```python
from build123d import *

# Parameters (mm, degrees)
BOSS_EXTRUDE1_DEPTH = 50.8
SKETCH2_W           = 479.425
SKETCH2_H           = 271.4625
CUT_EXTRUDE1_DEPTH  = 6.35
CUT_EXTRUDE2_DEPTH  = 762
SKETCH6_W           = 198.4375
SKETCH6_H           = 164.295373215
CUT_EXTRUDE3_DEPTH  = 10.922


with BuildPart() as part:
    # Sketch1 → Boss-Extrude1 (new body)
    with BuildSketch(Plane.XY):
        with BuildLine():
            Line((-255.5875, -170.65625), (255.5875, -170.65625))
            ThreePointArc((255.5875, -170.65625), (269.057884182, -165.076634182), (274.6375, -151.60625))
            Line((274.6375, -151.60625), (274.6375, 151.60625))
            ThreePointArc((274.6375, 151.60625), (269.057884182, 165.076634182), (255.5875, 170.65625))
            Line((255.5875, 170.65625), (-255.5875, 170.65625))
            ThreePointArc((-255.5875, 170.65625), (-269.057884182, 165.076634182), (-274.6375, 151.60625))
            Line((-274.6375, 151.60625), (-274.6375, -151.60625))
            ThreePointArc((-274.6375, -151.60625), (-269.057884182, -165.076634182), (-255.5875, -170.65625))
        make_face()
    extrude(amount=-BOSS_EXTRUDE1_DEPTH)

    # Sketch2 → Cut-Extrude1 (cut)
    with BuildSketch(Plane.XY):
        Rectangle(SKETCH2_W, SKETCH2_H)
    extrude(amount=-CUT_EXTRUDE1_DEPTH, mode=Mode.SUBTRACT)

    # Sketch4 → Cut-Extrude2 (cut)
    with BuildSketch(Plane(origin=(274.6375, 0, 0), x_dir=(0, 0, -1), z_dir=(1, 0, 0))):
        with BuildLine():
            Line((50.8, 151.60625), (24.619980511, 151.60625))
            add(Edge.make_bspline(
                [(24.619980511, 151.60625), (37.620188453, 124.390887767), (37.919518366, 93.154889178), (39.820271532, 62.244773812)],
                knots=[0.12550099, 0.12550099, 0.12550099, 0.12550099, 0.642402298, 0.642402298, 0.642402298, 0.642402298], degree=3))
            ThreePointArc((39.820271532, 62.244773812), (41.808148642, 58.008646197), (46.158299596, 56.284517648))
            Line((46.158299596, 56.284517648), (50.8, 56.284517648))
            Line((50.8, 56.284517648), (50.8, 151.60625))
        make_face()
        with BuildLine():
            Line((50.8, 170.65625), (12.7, 170.65625))
            add(Edge.make_bspline(
                [(12.7, 170.65625), (17.558504138, 164.584737247), (21.463596597, 158.21400058), (24.619980511, 151.60625)],
                knots=[0, 0, 0, 0, 0.12550099, 0.12550099, 0.12550099, 0.12550099], degree=3))
            Line((24.619980511, 151.60625), (50.8, 151.60625))
            Line((50.8, 151.60625), (50.8, 170.65625))
        make_face()
        with BuildLine():
            Line((50.8, -96.115482352), (50.8, -170.65625))
            Line((50.8, -170.65625), (12.7, -170.65625))
            add(Edge.make_bspline(
                [(12.7, -170.65625), (29.115546881, -150.814752865), (38.270494448, -127.771718295), (39.954605231, -102.050599403)],
                knots=[0, 0, 0, 0, 0.929133929, 0.929133929, 0.929133929, 0.929133929], degree=3))
            ThreePointArc((39.954605231, -102.050599403), (41.950070115, -97.830991726), (46.291037361, -96.115482352))
            Line((46.291037361, -96.115482352), (50.8, -96.115482352))
        make_face()
    extrude(amount=-CUT_EXTRUDE2_DEPTH, mode=Mode.SUBTRACT)

    # Sketch6 → Cut-Extrude3 (cut)
    with BuildSketch(Plane(origin=(0, 0, -50.8), x_dir=(-1, 0, 0), z_dir=(0, 0, -1))):
        with Locations((-175.41875, -19.902912796)):
            Rectangle(SKETCH6_W, SKETCH6_H)
        with Locations((175.41875, -19.902912796)):
            Rectangle(SKETCH6_W, SKETCH6_H)
    extrude(amount=-CUT_EXTRUDE3_DEPTH, mode=Mode.SUBTRACT)


solid = part.part
```
Can you work these out from the model? Positions are in its coordinate system, mm. Coordinates: 2 decimals unless noted, no trailing zeros. Loops run counter-clockwise (first coordinate to the right, second up) from the corner with the lowest first, then second, coordinate; pieces in that order, holes last. Notation, with made-up numbers: (19.5, -9.75) - (55.5, -9.75) arc R32 cw to (55.5, 22.25) - close; hole circle Ø7 at (35, 76). An arc over 180 degrees is marked (long way). Answer as CSV lines item,"result". Start each with the question number.
1) Suppose I cut it at A-A (y = -11). Please give me the cut outline in (x, z).
2) For pin 1 (4 mm diameter, centred on x = 213, y = 14, fed in from +Z); pin 2 (5 mm diameter, centred on x = -4.5, z = -48, fed in from +Y); pin 3 (4 mm diameter, centred on x = -87, y = -95.5, fed in from -Z), each with a flat end and sliding along its axis, tell me the tip position at first contact or that it passes through.
3) I need wall thicknesses on line 1 (Y direction, x = 123, z = -1.5); line 2 (Z direction, x = -20, y = -89); line 3 (Z direction, x = 230, y = 39). Which ranges of each line are inside material? Lowest first, please. Write a range as from..to.
4) Thinking about a two-plate mould opening in Y: for faces 1 (the cylindrical face through (271.071, -162.704, -9.813)), 2 (the flat face through (-274.638, 2, -20)), 3 (the flat face through (-3, 2, -6.35)), which applies, pulls with the +Y half, pulls with the -Y half, needs draft (parallel to the pull), parting line crosses it, or undercut?
Check result:
1,outline,"(-274.64, -39.88) - (-76.2, -39.88) - (-76.2, -50.8) - (76.2, -50.8) - (76.2, -39.88) - (274.64, -39.88) - (274.64, 0) - (239.71, 0) - (239.71, -6.35) - (-239.71, -6.35) - (-239.71, 0) - (-274.64, 0) - close"
2,pin 1,"stops at z = -6.35"
2,pin 2,"stops at y = 56.32"
2,pin 3,"stops at z = -39.88"
3,line 1,"y = -170.66..-135.73, 135.73..170.66"
3,line 2,"z = -50.8..-6.35"
3,line 3,"z = -39.88..-6.35"
4,face 1,"pulls with the -Y half"
4,face 2,"needs draft"
4,face 3,"undercut"
